Could you check a few things on this drawing? It's one solid part, dimensions in mm from its lowest x, y, z. A direction names the side the tool comes from. Round coordinates to 2 decimals unless told otherwise and drop trailing zeros. Loops run counter-clockwise (first coordinate to the right, second up) from the corner with the lowest first, then second, coordinate; pieces in that order, holes last. Notation, with made-up numbers: (55.25, -1.75) -> (104.25, -1.75) arc R28 cw to (104.25, 25.25) -> close; hole circle Ø9 at (43, 83). An arc over 180 degrees is marked (long way). Put each result on its own line as item: value. Start each with the question number.
1. Imagine slicing it at B-B, the plane y = 2.75. Please give me the cut outline in (x, z), and give its area (3 significant figures).
2. Imagine slicing it at D-D, the plane x = 107.5. Please give me the cut outline in (y, z).
3. Imagine slicing it at A-A, the plane x = 17.5. Please give me the cut outline in (y, z).
4. Imagine slicing it at C-C, the plane z = 57.5. Please give me the cut outline in (x, y).
5. I'm going to push flat-ended pins straight in: P1, Ø10.5, axis at x = 7.5, z = 107.5, coming from the -Y side; P2, Ø4, axis at x = 97.5, z = 54, coming from the +Y side; P3, Ø2.5, axis at x = 7.5, z = 7.5, coming from the -Y side; P4, Ø2.5, axis at y = 5, z = 58, coming from the +X side. Where does each tip first touch, or does it pass through?
6. Which directions (+Z, -Z, +X, -X, +Y, -Y) give clear straight access to the entire face, cutting with the end or side of a thin tool? Please do the marked faces 1 and 2.
7. I need wall thicknesses on line 1 (Z direction, x = 7.5, y = 14.15); line 2 (Z direction, x = 107.5, y = 21.15); line 3 (Y direction, x = 80, z = 81.5). Which ranges of each line are inside material? Lowest first, please. Write a range as [from, to].
8. If we mould it in two halves opening along Y, with no side actions, what happens to the marked faces 3 and 4? For each: pulls with the +Y half, pulls with the -Y half, needs draft (parallel to the pull), parting line crosses it, or undercut.
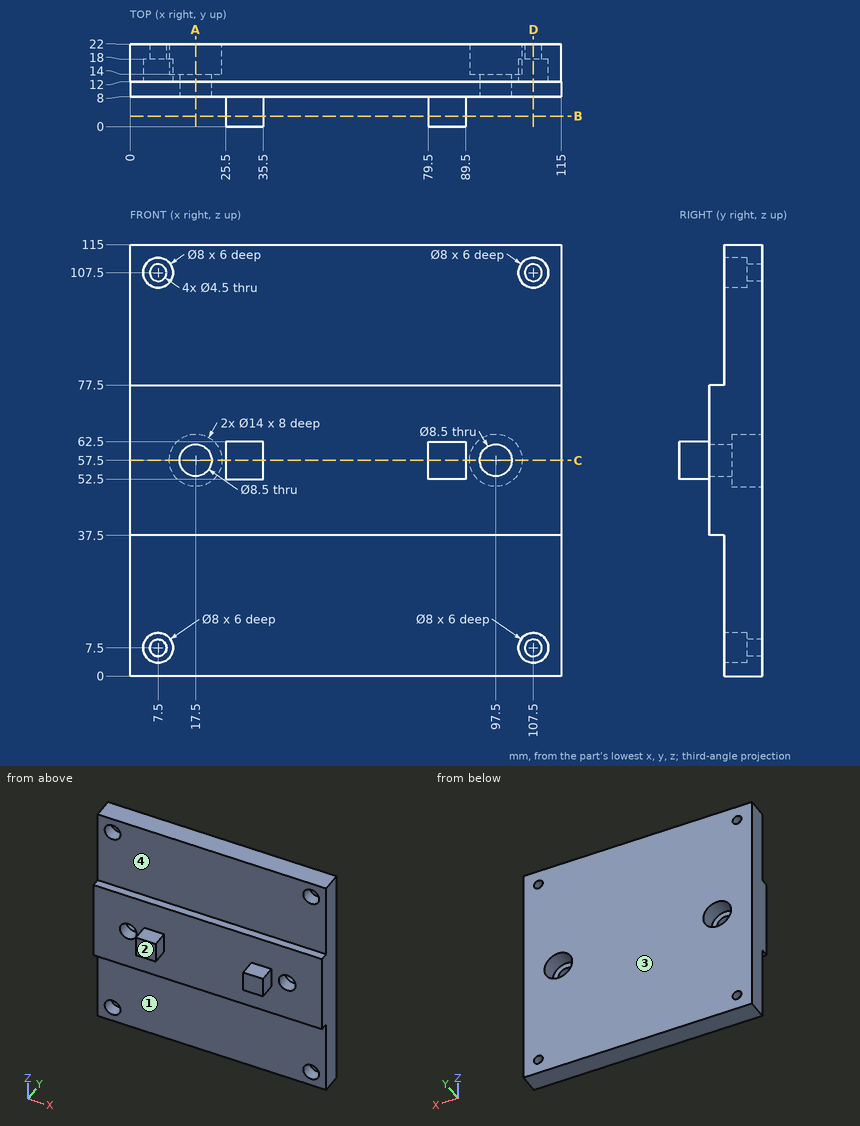
Entries:
1. outline: (25.5, 52.5) -> (35.5, 52.5) -> (35.5, 62.5) -> (25.5, 62.5) -> close; (79.5, 52.5) -> (89.5, 52.5) -> (89.5, 62.5) -> (79.5, 62.5) -> close
1. area: 200 mm^2
2. outline: (8, 37.5) -> (12, 37.5) -> (12, 11.5) -> (18, 11.5) -> (18, 9.75) -> (22, 9.75) -> (22, 105.25) -> (18, 105.25) -> (18, 103.5) -> (12, 103.5) -> (12, 77.5) -> (8, 77.5) -> close; (12, 0) -> (22, 0) -> (22, 5.25) -> (18, 5.25) -> (18, 3.5) -> (12, 3.5) -> close; (12, 111.5) -> (18, 111.5) -> (18, 109.75) -> (22, 109.75) -> (22, 115) -> (12, 115) -> close
3. outline: (8, 37.5) -> (12, 37.5) -> (12, 0) -> (22, 0) -> (22, 50.5) -> (14, 50.5) -> (14, 53.25) -> (8, 53.25) -> close; (8, 61.75) -> (14, 61.75) -> (14, 64.5) -> (22, 64.5) -> (22, 115) -> (12, 115) -> (12, 77.5) -> (8, 77.5) -> close
4. outline: (0, 8) -> (13.25, 8) -> (13.25, 14) -> (10.5, 14) -> (10.5, 22) -> (0, 22) -> close; (21.75, 8) -> (25.5, 8) -> (25.5, 0) -> (35.5, 0) -> (35.5, 8) -> (79.5, 8) -> (79.5, 0) -> (89.5, 0) -> (89.5, 8) -> (93.25, 8) -> (93.25, 14) -> (90.5, 14) -> (90.5, 22) -> (24.5, 22) -> (24.5, 14) -> (21.75, 14) -> close; (101.75, 8) -> (115, 8) -> (115, 22) -> (104.5, 22) -> (104.5, 14) -> (101.75, 14) -> close
5. P1: y = 12
5. P2: y = 14
5. P3: through
5. P4: x = 89.5
6. face 1: -Z, +X, -X, -Y
6. face 2: +Z, -Z, +X, -X, -Y
7. line 1: [0, 3.5], [11.5, 103.5], [111.5, 115]
7. line 2: [0, 5.25], [9.75, 105.25], [109.75, 115]
7. line 3: [12, 22]
8. face 3: pulls with the +Y half
8. face 4: pulls with the -Y half
